from build123d import *

# Parameters (mm, degrees)
F1_DEPTH     = 14.0906665474
F3_D         = 45.72
F4_R         = 6.858
F5_T4_DEPTH  = 103.1253973126
F5_S5_R      = 27.6648668559
F5_T6_DEPTH  = 53
F5_T10_DEPTH = 103.1253973126
F5_S11_R     = 27.6648668559
F5_T12_DEPTH = 53


# Not quite as in the source:
# - a fillet or chamfer that OpenCascade refuses, or shapes differently, is made with other operations: its cross-section is extruded or revolved along the edge and cut away or added


with BuildPart() as f1:
    # F0 (on Front) → F1 (new body)
    with BuildSketch(Plane.XZ):
        with BuildLine():
            ThreePointArc((26.2165333562, -8.9155114296), (27.3140546761, -4.5315667493), (27.6831785203, -0.0274273648))
            ThreePointArc((27.6831785203, -0.0274273648), (27.3786909177, 4.0657993906), (26.4719306688, 8.0689236483))
            Line((26.4719306688, 8.0689236483), (-26.4353073399, 8.0689236483))
            Line((-26.4353073399, 8.0689236483), (-26.4353073399, -8.1237783779))
            ThreePointArc((-26.4353073399, -8.1237783779), (-26.3105848654, -8.5206049607), (-26.1799100273, -8.9155114296))
            Line((-26.1799100273, -8.9155114296), (26.2165333562, -8.9155114296))
        make_face()
        with BuildLine():
            ThreePointArc((26.4719306688, 8.0689236483), (27.3786909177, 4.0657993906), (27.6831785203, -0.0274273648))
            ThreePointArc((27.6831785203, -0.0274273648), (27.3140546761, -4.5315667493), (26.2165333562, -8.9155114296))
            Line((26.2165333562, -8.9155114296), (59.9537639373, -8.9155114296))
            Line((59.9537639373, -8.9155114296), (60.1102084538, 8.0689236483))
            Line((60.1102084538, 8.0689236483), (26.4719306688, 8.0689236483))
        make_face()
        with BuildLine():
            Line((-26.4353073399, 8.0689236483), (26.4719306688, 8.0689236483))
            ThreePointArc((26.4719306688, 8.0689236483), (0.0183116645, 27.6374394911), (-26.4353073399, 8.0689236483))
        make_face()
        with BuildLine():
            ThreePointArc((-26.1799100273, -8.9155114296), (0.0183116645, -27.6922942207), (26.2165333562, -8.9155114296))
            Line((26.2165333562, -8.9155114296), (-26.1799100273, -8.9155114296))
        make_face()
        with BuildLine():
            Line((-26.4353073399, -8.1237783779), (-26.4353073399, 8.0689236483))
            ThreePointArc((-26.4353073399, 8.0689236483), (-27.6465551914, -0.0274273648), (-26.4353073399, -8.1237783779))
        make_face()
        with BuildLine():
            Line((-26.4353073399, -8.9155114296), (-26.1799100273, -8.9155114296))
            ThreePointArc((-26.1799100273, -8.9155114296), (-26.3105848654, -8.5206049607), (-26.4353073399, -8.1237783779))
            Line((-26.4353073399, -8.1237783779), (-26.4353073399, -8.9155114296))
        make_face()
    extrude(amount=F1_DEPTH)

    # F3 (through all)
    with Locations(Plane(origin=(0, 0, 0), x_dir=(1, 0, 0), z_dir=(0, 1, 0))):
        with Locations((0, 0)):
            Hole(F3_D / 2)

    # F4
    f4_edges = [f1.edges().sort_by_distance(p)[0] for p in [
        (43.085149, -14.090667, -8.915511),
        (43.085149, 0, -8.915511),
        (43.29107, -14.090667, 8.068924),
        (43.29107, 0, 8.068924),
    ]]
    fillet(f4_edges, radius=F4_R)

    # F5: fillet of radius 6.858 on 2 edges, made by hand


with BuildPart() as f5_tool2:
    # F5_s3 → F5_t4 (new body)
    with BuildSketch(Plane.YZ.offset(-43.5803073399)):
        with BuildLine():
            ThreePointArc((-14.0906665474, -2.0575114296), (-12.0820048528, -6.906849735), (-7.2326665474, -8.9155114296))
            Line((-7.2326665474, -8.9155114296), (-14.0906665474, -8.9155114296))
            Line((-14.0906665474, -8.9155114296), (-14.0906665474, -2.0575114296))
        make_face()
    extrude(amount=F5_T4_DEPTH)

    # F5_s5 → F5_t6 (cut, symmetric)
    with BuildSketch(Plane.XZ.offset(10.7)):
        with Locations((0.0183116645, -0.0274273648)):
            Circle(F5_S5_R)
    extrude(amount=F5_T6_DEPTH, both=True, mode=Mode.SUBTRACT)


with BuildPart() as f1_1:
    add(f1.part)

    # F5_t1: cut F5_tool2
    add(f5_tool2.part, mode=Mode.SUBTRACT)


with BuildPart() as f5_tool8:
    # F5_s9 → F5_t10 (new body)
    with BuildSketch(Plane.YZ.offset(-43.5803073399)):
        with BuildLine():
            ThreePointArc((0, -2.0575114296), (-2.0086616946, -6.906849735), (-6.858, -8.9155114296))
            Line((-6.858, -8.9155114296), (0, -8.9155114296))
            Line((0, -8.9155114296), (0, -2.0575114296))
        make_face()
    extrude(amount=F5_T10_DEPTH)

    # F5_s11 → F5_t12 (cut, symmetric)
    with BuildSketch(Plane.XZ.offset(3.4)):
        with Locations((0.0183116645, -0.0274273648)):
            Circle(F5_S11_R)
    extrude(amount=F5_T12_DEPTH, both=True, mode=Mode.SUBTRACT)


with BuildPart() as f1_2:
    add(f1_1.part)

    # F5_t7: cut F5_tool8
    add(f5_tool8.part, mode=Mode.SUBTRACT)


solid = f1_2.part
Can you work these out from the model? Positions are in its coordinate system, mm. A direction names the side the tool comes from. Coordinates: 2 decimals unless noted, no trailing zeros. Write each loop counter-clockwise with the first axis right and the second up, starting at its lowest first coordinate (ties: lowest second). Pieces come first, ordered by that corner, then holes.
Q1. Which directions (+Z, -Z, +X, -X, +Y, -Y) give clear straight access to the entire face, cutting with the end or side of a thin tool? Please do faces 3 (the face through (43.06, -1.96, 6.01)), 4 (the face through (22.5, 0, 6.2)), 5 (the face through (43.35, -2.06, -6.96)), 6 (the face through (43.35, -12.03, -6.96)).
Results found:
face 3: +Z, +X, +Y
face 4: +Z, -Z, +X, -X, +Y
face 5: -Z, +X, +Y
face 6: -Z, +X, -Y
Q2. Please list where these lines run through material, in increasing order: L1, parallel to Z at x = 0, y = -8; L2, parallel to Z at x = 49, y = -7; L3, parallel to X at y = -1.25, z = -14.
Results found:
L1: z = -27.69 to -22.86, 22.86 to 27.64
L2: z = -8.92 to 8.07
L3: x = -23.86 to -18.07, 18.07 to 23.9
Q3. Imagine slicing it at A-A, the plane x = 0. List the corners of the cut face in (y, z) for me.
Results found:
outline: (-14.09, -27.69) - (0, -27.69) - (0, -22.86) - (-14.09, -22.86) - close; (-14.09, 22.86) - (0, 22.86) - (0, 27.64) - (-14.09, 27.64) - close
Q4. Imagine slicing it at B-B, the plane z = 0. List the corners of the cut face in (x, y) for me, plus the area to 3 significant figures.
Results found:
outline: (-27.65, -14.09) - (-22.86, -14.09) - (-22.86, 0) - (-27.65, 0) - close; (22.86, -14.09) - (60.04, -14.09) - (60.04, 0) - (22.86, 0) - close
area: 591 mm2
Q5. If we mould it in two halves opening along X, with no side actions, what happens to faces 1 (the face through (43.056, -12.135, 6.007)), 2 (the face through (-21.804, -7.144, -6.867))? For each: +X half, -X half, draft (parallel to the pull), parting line (faces both ways), or undercut.
Results found:
face 1: draft
face 2: undercut
Q6. For P1, Ø5, axis at x = -16.5, y = -11.5, coming from the -Z side; P2, Ø5, axis at y = -10.5, z = 16, coming from the -X side; P3, Ø1, axis at x = 3, y = -3.5, coming from the +Z side, each with a flat end and sliding along its axis, tell me the tip position at first contact or that it passes through.
Results found:
P1: stops at z = -23.88
P2: stops at x = -24.11
P3: stops at z = 27.53
Q7. Imagine slicing it at D-D, the plane x = 46. List the corners of the cut face in (y, z) for me, plus the area to 3 significant figures.
Results found:
outline: (-14.09, -2.06) arc R6.86 ccw to (-7.23, -8.92) - (-6.86, -8.92) arc R6.86 ccw to (0, -2.06) - (0, 1.21) arc R6.86 ccw to (-6.86, 8.07) - (-7.23, 8.07) arc R6.86 ccw to (-14.09, 1.21) - close
area: 199 mm2
